```python
from build123d import *

# Parameters (mm, degrees)
F1_DEPTH    = 3
F2_SIZE     = 0.5
F3_R        = 2.2
F4_DEPTH    = 1.5
F5_R        = 1
F6_DEPTH    = 25
F7_T2_ANGLE = 66.979105944
F7_T4_ANGLE = 66.979105944
F9_START    = -1
F9_DEPTH    = 1


# Not quite as in the source:
# - a fillet or chamfer that OpenCascade refuses, or shapes differently, is made with other operations: its cross-section is extruded or revolved along the edge and cut away or added


with BuildPart() as f1:
    # F0 (on Right) → F1 (new body)
    with BuildSketch(Plane.YZ):
        with BuildLine():
            ThreePointArc((0, -2), (1.4142135624, -1.4142135624), (2, 0))
            ThreePointArc((2, 0), (1.4142135624, 1.4142135624), (0, 2))
            ThreePointArc((0, 2), (-2, 0), (0, -2))
        make_face()
        with BuildLine():
            ThreePointArc((0, -2), (-2, 0), (0, 2))
            ThreePointArc((0, 2), (-3.6215795528, 2.5039519212), (-6.9679827429, 3.9775162004))
            ThreePointArc((-6.9679827429, 3.9775162004), (-5.2841991645, -8.562454479), (-12.0608618515, -19.247155439))
            ThreePointArc((-12.0608618515, -19.247155439), (-27.2940486142, -42.4780574149), (-24.8540620048, -70.1506295922))
            ThreePointArc((-24.8540620048, -70.1506295922), (-24.9977932498, -60.4898051339), (-22.5043967366, -51.1551834643))
            ThreePointArc((-22.5043967366, -51.1551834643), (-23.2047477115, -50.1129852075), (-23.3636565752, -48.8674264303))
            ThreePointArc((-23.3636565752, -48.8674264303), (-18.817838904, -34.5662944148), (-9.0101721364, -23.2086314596))
            ThreePointArc((-9.0101721364, -23.2086314596), (-1.7247742588, -13.7854899156), (0, -2))
        make_face()
    extrude(amount=F1_DEPTH)

    # F2
    f2_edges = [f1.edges().sort_by_distance(p)[0] for p in [
        (3, 2, 0),
        (3, -3.62158, 2.503952),
        (3, -5.284199, -8.562454),
        (3, -27.294049, -42.478057),
        (3, -24.997793, -60.489805),
        (3, -23.204748, -50.112985),
        (3, -18.817839, -34.566294),
        (3, -1.724774, -13.78549),
        (0, 2, 0),
        (0, -3.62158, 2.503952),
        (0, -5.284199, -8.562454),
        (0, -27.294049, -42.478057),
        (0, -24.997793, -60.489805),
        (0, -23.204748, -50.112985),
        (0, -18.817839, -34.566294),
        (0, -1.724774, -13.78549),
    ]]
    chamfer(f2_edges, length=F2_SIZE)

    # F3 (on face) → F4 (cut)
    with BuildSketch(Plane.YZ.offset(3)):
        Circle(F3_R)
    extrude(amount=-F4_DEPTH, mode=Mode.SUBTRACT)

    # F5 (on face) → F6 (cut)
    with BuildSketch(Plane.YZ.offset(1.5)):
        Circle(F5_R)
    extrude(amount=-F6_DEPTH, mode=Mode.SUBTRACT)

    # F7: chamfer of 2.5 on 2 edges, made by hand

    # F7_s1 → F7_t2 (revolve, cut)
    with BuildSketch(Plane(origin=(0, 33.2597277938, -48.8887943232), x_dir=(1, 0, 0), z_dir=(0, 0.5624874969, -0.8268057909))):
        Polygon((0, 66.4232158642), (1.767766953, 62.1554489112), (0, 63.9232158642), align=None)
    revolve(axis=Axis((0, 9.8679252657, -64.8025634284), (-1, 0, 0)), revolution_arc=F7_T2_ANGLE, mode=Mode.SUBTRACT)

    # F7_s3 → F7_t4 (revolve, cut)
    with BuildSketch(Plane(origin=(0, 33.2597277938, -48.8887943232), x_dir=(1, 0, 0), z_dir=(0, 0.5624874969, -0.8268057909))):
        Polygon((3, 66.4232158642), (1.232233047, 62.1554489112), (3, 63.9232158642), align=None)
    revolve(axis=Axis((3, 9.8679252657, -64.8025634284), (-1, 0, 0)), revolution_arc=F7_T4_ANGLE, mode=Mode.SUBTRACT)

    # F8 (on face) → F9 (cut)
    with BuildSketch(Plane.YZ.offset(3).offset(F9_START)):
        with BuildLine():
            ThreePointArc((14, 0), (0, 14), (-14, 0))
            ThreePointArc((-14, 0), (0, -14), (14, 0))
        make_face()
        with BuildLine():
            ThreePointArc((-12, 0), (0, 12), (12, 0))
            ThreePointArc((12, 0), (0, -12), (-12, 0))
        make_face(mode=Mode.SUBTRACT)
    extrude(amount=-F9_DEPTH, mode=Mode.SUBTRACT)


solid = f1.part
```
The listing builds one solid part. Answer for the finished solid, in the listing's coordinates (mm). A direction names the side the tool comes from. Give positions to 0.01 mm unless a question says otherwise; leave off trailing zeros.
1) Consider line 1 along Z through (x, y) = (1.85, -10.5); line 2 along Y through (x, z) = (2.1, -21); line 3 along Y through (x, z) = (1.7, -40). Determine where each line is inside the solid, lowest interval first.
Reported:
line 1: z = -24.42 to -17.9
line 2: y = -14.19 to -6.53
line 3: y = -26.59 to -21.31
2) For faces 1 (the face through (1, -4, -12)), 2 (the face through (1.507, -3.471, -11.487)), 3 (the face through (0.768, -25.336, -56.043)), 4 (the face through (2.232, -25.336, -56.043)), determine the directions among +Z, -Z, +X, -X, +Y, -Y from which every point of the face is accessible in a straight line to the end or side of a thin tool.
Reported:
face 1: none
face 2: -Y
face 3: -X, +Y
face 4: +X, +Y
3) Determine the mould class of faces 5 (the face through (3, -14, -25)), 6 (the face through (1, 0, -1)), 7 (the face through (1.486, -27.196, -42.094)) for opening direction Z: pulls with the +Z half, pulls with the -Z half, needs draft (parallel to the pull), parting line crosses it, or undercut.
Reported:
face 5: needs draft
face 6: undercut
face 7: parting line crosses it
